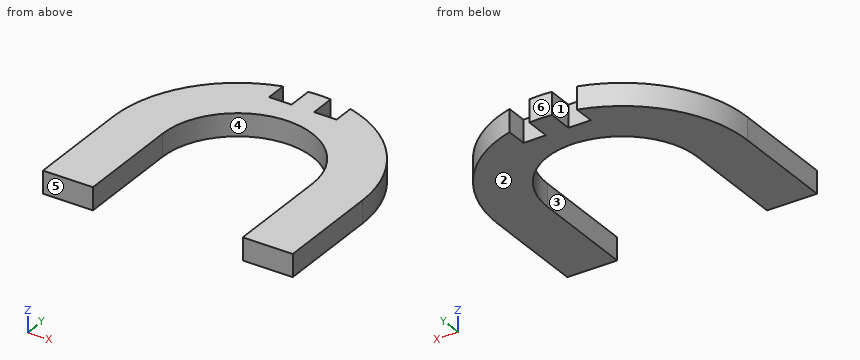
from build123d import *

# Parameters (mm, degrees)
BOSS_EXTRUDE1_DEPTH = 18
SKETCH2_W           = 18
SKETCH2_H           = 46.670060525
CUT_EXTRUDE1_DEPTH  = 19
SKETCH3_W           = 40
SKETCH3_H           = 18
BOSS_EXTRUDE2_DEPTH = 44


with BuildPart() as part:
    # Sketch1 → Boss-Extrude1 (new body)
    with BuildSketch(Plane.XY):
        with BuildLine():
            Line((60, 60), (60, 100.646547639))
            ThreePointArc((60, 100.646547639), (0, 160.646547639), (-60, 100.646547639))
            Line((-60, 100.646547639), (-60, 60))
            Line((-60, 60), (-100, 60))
            Line((-100, 60), (-100, 100.646547639))
            ThreePointArc((-100, 100.646547639), (0, 200.646547639), (100, 100.646547639))
            Line((100, 100.646547639), (100, 60))
            Line((100, 60), (60, 60))
        make_face()
    extrude(amount=BOSS_EXTRUDE1_DEPTH)

    # Sketch2 → Cut-Extrude1 (cut, through all)
    with BuildSketch(Plane.XY.offset(18)):
        with Locations((18, 203.335030263)):
            Rectangle(SKETCH2_W, SKETCH2_H)
        with Locations((-18, 203.335030263)):
            Rectangle(SKETCH2_W, SKETCH2_H)
    extrude(amount=-CUT_EXTRUDE1_DEPTH, mode=Mode.SUBTRACT)

    # Sketch3 → Boss-Extrude2 (add)
    with BuildSketch(Plane.XZ.offset(-60)):
        with Locations((-80, 9)):
            Rectangle(SKETCH3_W, SKETCH3_H)
        with Locations((80, 9)):
            Rectangle(SKETCH3_W, SKETCH3_H)
    extrude(amount=BOSS_EXTRUDE2_DEPTH)


solid = part.part
For this review, take the finished solid that the model builds, in its own axes (mm). Face numbers are marked on the shaded views. A direction names the side the tool comes from. Round coordinates to 2 decimals unless told otherwise and drop trailing zeros. Order: outer loops, then holes, each group sorted by start corner. A loop starts at its lowest first (then second) coordinate and runs counter-clockwise, first axis right, second up. Notation, with made-up numbers: M 29,32 L 85,32 A12 ccw 85,37 Z; hole C -34.5,-18 d8. An arc over 180 degrees is marked long. Write each question's results on one line, items separated by ' | '. Start each with the question number.
1. To check wall thickness, follow L1, parallel to X at y = 63.5, z = 6.25; L2, parallel to X at y = 189, z = 8.5; L3, parallel to X at y = 149.5, z = 5.25. State the ranges of each line that lie inside material, in increasing order. Write a range as [from, to].
2. Add section B-B (z = 5.5). State the section outline as (x, y) points, then the cut area to 3 significant figures.
3. Add section C-C (x = 0). State the section outline as (y, z) points.
4. Tool access review of the marked faces 1, 2 and 3: name each direction out of +Z, -Z, +X, -X, +Y, -Y from which nothing blocks a thin tool from reaching the whole face with its end or side.
5. Add section A-A (y = 47). State the section outline as (x, z) points.
6. Add section D-D (x = -36.5). State the section outline as (y, z) points, then the cut area to 3 significant figures.
7. Draft analysis for pull direction X (two halves, no side actions). For the marked faces 4, 5 and 6, state which applies: pulls with the +X half, pulls with the -X half, needs draft (parallel to the pull), parting line crosses it, or undercut.
8. Clearance check with flat-ended pins moving along their axes: pin 1 Ø12 at (x, y) = (76.5, 99.5) entering from -Z; pin 2 Ø9 at (y, z) = (186.5, 11) entering from +X; pin 3 Ø5 at (y, z) = (136, 6.5) entering from +X; pin 4 Ø5.5 at (y, z) = (194.5, 6.5) entering from -X. State where each tip first meets the part, or that it passes through.
Output values:
1) L1: [-100, -60], [60, 100] | L2: [-46.84, -27], [-9, 9], [27, 46.84] | L3: [-87.25, -34.83], [34.83, 87.25]
2) outline: M -100,16 L -60,16 L -60,100.65 A60 cw 60,100.65 L 60,16 L 100,16 L 100,100.65 A100 ccw 27,196.93 L 27,180 L 9,180 L 9,200.24 A100 ccw -9,200.24 L -9,180 L -27,180 L -27,196.93 A100 ccw -100,100.65 Z | area: 16,100 mm^2
3) outline: M 160.65,0 L 200.65,0 L 200.65,18 L 160.65,18 Z
4) face 1: +Z, -Z, +Y | face 2: -Z, +X, -X, +Y, -Y | face 3: +Z, -Z, -Y
5) outline: M -100,0 L -60,0 L -60,18 L -100,18 Z; M 60,0 L 100,0 L 100,18 L 60,18 Z
6) outline: M 148.27,0 L 193.75,0 L 193.75,18 L 148.27,18 Z | area: 819 mm^2
7) face 4: undercut | face 5: needs draft | face 6: parting line crosses it
8) pin 1: z = 0 | pin 2: x = 58.15 | pin 3: x = 94.45 | pin 4: x = -41.23
